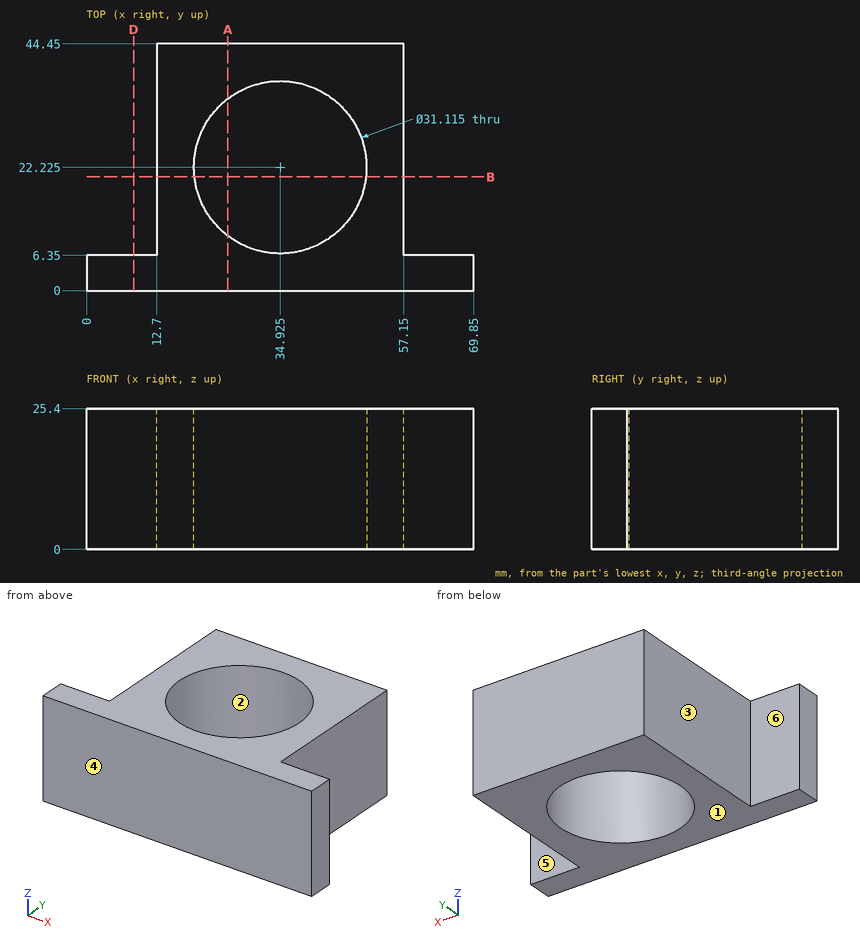
Answer from the drawing. Dimensions are ordinates in mm from the lowest x, y and z of the part. A direction names the side the tool comes from. Coordinates: 2 decimals unless noted, no trailing zeros. Write each loop counter-clockwise with the first axis right and the second up, starting at its lowest first coordinate (ties: lowest second). Pieces come first, ordered by that corner, then holes. Notation, with made-up numbers: M -40,17 L -36,17 A17 ccw -36,40 Z; hole C 62,67 d1. An arc over 180 degrees is marked long. Use one line per item in the form item = value. Start each with the question number.
1. The part is cut by section A-A (x = 25.5). Give the vertices of the cut face in (y, z).
2. Each of these flat-tipped pins is pushed along its axis until it touches: P1, Ø14, axis at x = 5.5, z = 9.5, coming from the +Y side; P2, Ø3, axis at y = 7, z = 15, coming from the -X side; P3, Ø12, axis at y = 32.5, z = 21.5, coming from the +X side; P4, Ø12.5, axis at y = 35, z = 17.5, coming from the -X side. Where does it stop, or does it pass through?
3. The mould has two halves that part along X. Classify the marked faces 1, 2 and 3: released by +X, released by -X, zero draft, split by the parting line, or undercut.
4. The part is cut by section D-D (x = 8.5). Give the vertices of the cut face in (y, z).
5. Straight lines are drawn through the part: probe 1 along Y at (x, z) = (65, 15.5); probe 2 along X at (y, z) = (27, 5); probe 3 along X at (y, z) = (23, 23.5). For each, find the intervals that lie inside material, in ascending order. Write a range as from..to.
6. The part is cut by section B-B (y = 20.5). Give the vertices of the cut face in (x, z), plus the area to 3 significant figures.
7. A tool of negligible diameter and unlimited length cuts with its end or side. For the marked faces 4, 5 and 6, from which of +Z, -Z, +X, -X, +Y, -Y can it reach the whole face along a straight path? Write none if from no direction.
Evaluation:
q1.outline = M 0,0 L 9.85,0 L 9.85,25.4 L 0,25.4 Z; M 34.6,0 L 44.45,0 L 44.45,25.4 L 34.6,25.4 Z
q2.P1 = 6.35
q2.P2 = 0
q2.P3 = 57.15
q2.P4 = 12.7
q3.face_1 = zero draft
q3.face_2 = undercut
q3.face_3 = released by -X
q4.outline = M 0,0 L 6.35,0 L 6.35,25.4 L 0,25.4 Z
q5.probe_1 = 0..6.35
q5.probe_2 = 12.7..20.12, 49.73..57.15
q5.probe_3 = 12.7..19.39, 50.46..57.15
q6.outline = M 12.7,0 L 19.46,0 L 19.46,25.4 L 12.7,25.4 Z; M 50.39,0 L 57.15,0 L 57.15,25.4 L 50.39,25.4 Z
q6.area = 344 mm^2
q7.face_4 = +Z, -Z, +X, -X, -Y
q7.face_5 = +Z, -Z, +X, +Y
q7.face_6 = +Z, -Z, -X, +Y
